from build123d import *

# Parameters (mm, degrees)
BOSS_EXTRUDE1_DEPTH = 1.5875
SKETCH2_W           = 192.0875
SKETCH2_H           = 15.875
CUT_EXTRUDE1_DEPTH  = 1.5875
SKETCH4_R           = 3.2639
CUT_EXTRUDE2_DEPTH  = 9.906
SKETCH5_W           = 250.81556442
SKETCH5_H           = 138.767374129
CUT_EXTRUDE3_DEPTH  = 125.222


with BuildPart() as part:
    # Sketch1 → Boss-Extrude1 (new body)
    with BuildSketch(Plane(origin=(0, 0, 0), x_dir=(1, 0, 0), z_dir=(0, 1, 0))):
        Polygon((-96.04375, 177.8), (35.321875, 177.8), (35.321875, 145.036189145), (78.58125, 145.036189145), (78.58125, 177.8), (96.04375, 177.8), (96.04375, -177.8), (-96.04375, -177.8), align=None)
    extrude(amount=BOSS_EXTRUDE1_DEPTH)

    # Sketch2 → Cut-Extrude1 (cut)
    with BuildSketch(Plane(origin=(0, 1.5875, 0), x_dir=(1, 0, 0), z_dir=(0, 1, 0))):
        with Locations((0, -88.9)):
            Rectangle(SKETCH2_W, SKETCH2_H)
        Polygon((-78.58125, 177.8), (-96.04375, 139.7), (-96.04375, 177.8), align=None)
        Polygon((96.04375, 139.7), (78.58125, 177.8), (96.04375, 177.8), align=None)
    extrude(amount=-CUT_EXTRUDE1_DEPTH, mode=Mode.SUBTRACT)

    # Sketch4 → Cut-Extrude2 (cut)
    with BuildSketch(Plane(origin=(0, 1.5875, 0), x_dir=(1, 0, 0), z_dir=(0, 1, 0))):
        with Locations((33.07715, 87.20455)):
            Circle(SKETCH4_R)
        with Locations((-38.93185, 87.20455)):
            Circle(SKETCH4_R)
    extrude(amount=-CUT_EXTRUDE2_DEPTH, mode=Mode.SUBTRACT)

    # Sketch5 → Cut-Extrude3 (cut)
    with BuildSketch(Plane(origin=(0, 1.5875, 0), x_dir=(1, 0, 0), z_dir=(0, 1, 0))):
        with Locations((-21.956348657, -157.127502405)):
            Rectangle(SKETCH5_W, SKETCH5_H)
    extrude(amount=-CUT_EXTRUDE3_DEPTH, mode=Mode.SUBTRACT)


solid = part.part
Design review of the part built by this model. Coordinates are the model's own, in mm. Give positions to 0.01 mm unless a question says otherwise; leave off trailing zeros. Loops run counter-clockwise (first coordinate to the right, second up) from the corner with the lowest first, then second, coordinate; pieces in that order, holes last. Notation, with made-up numbers: (39.5, 57) - (66.5, 57) arc R13 cw to (66.5, 62) - close; hole circle Ø6 at (80, 31). An arc over 180 degrees is marked (long way). Use CSV: the item, a comma, the result in double quotes. Start each with the question number.
1. Add section A-A (y = 0.5). State the section outline as (x, z) points.
2. Add section B-B (z = -162). State the section outline as (x, y) points.
3. Insertion check: P1, Ø0.8, axis at x = 64.5, y = 1, coming from the -Z side; P2, Ø0.5, axis at y = 1, z = -155.5, coming from the -X side. Each pin has a flat end and moves straight along its axis. Give the tip position at first contact, or say it passes through.
4. Draft analysis for pull direction X (two halves, no side actions). For faces 1 (the flat face through (-87.2, 0.8, -159)), 2 (the cylindrical face through (34.583, 0.805, -84.309)), 3 (the flat face through (1, 0, -50)), state which applies: released by +X, released by -X, zero draft, split by the parting line, or undercut.
5. Add section C-C (x = 65). State the section outline as (y, z) points.
6. Wall thickness on L1, parallel to Z at x = -38.5, y = 0.7; L2, parallel to X at y = 1, z = -84.5; L3, parallel to Z at x = 55, y = 1: over which ranges is each line inside the solid? List them lowest first.
Results found:
1,outline,"(-96.04, -139.7) - (-78.58, -177.8) - (35.32, -177.8) - (35.32, -145.04) - (78.58, -145.04) - (78.58, -177.8) - (96.04, -139.7) - (96.04, 80.96) - (-96.04, 80.96) - close; hole circle Ø6.53 at (-38.93, -87.2); hole circle Ø6.53 at (33.08, -87.2)"
2,outline,"(-85.82, 0) - (35.32, 0) - (35.32, 1.59) - (-85.82, 1.59) - close; (78.58, 0) - (85.82, 0) - (85.82, 1.59) - (78.58, 1.59) - close"
3,P1,"stops at z = -145.04"
3,P2,"stops at x = -88.92"
4,face 1,"released by -X"
4,face 2,"undercut"
4,face 3,"zero draft"
5,outline,"(0, -145.04) - (1.59, -145.04) - (1.59, 80.96) - (0, 80.96) - close"
6,L1,"z = -177.8 to -90.44, -83.97 to 80.96"
6,L2,"x = -96.04 to -40.76, -37.1 to 31.25, 34.9 to 96.04"
6,L3,"z = -145.04 to 80.96"
